The model under review builds one solid part; all positions refer to its coordinate system, in mm. Face numbers are marked on the shaded views. Round coordinates to 2 decimals unless told otherwise and drop trailing zeros. Order: outer loops, then holes, each group sorted by start corner. A loop starts at its lowest first (then second) coordinate and runs counter-clockwise, first axis right, second up. Notation, with made-up numbers: (-33, 31.25) -> (5, 31.25) arc R12 cw to (5, 53.25) -> close; hole circle Ø11 at (13, 86.25). An arc over 180 degrees is marked (long way). Use a Markdown table: item, result. Add a question column.
```python
from build123d import *

# Parameters (mm, degrees)
SKETCH_1_R               = 25
EXTRUDE_2_DEPTH          = 1
SKETCH_2_R               = 1.5
CUT_EXTRUDE_1_DEPTH      = 1
PATTERN_CIRCULAR_1_COUNT = 8
CUT_EXTRUDE_2_DEPTH      = 1
EXTRUDE_3_DEPTH          = 1
SKETCH_5_R               = 25
EXTRUDE_5_DEPTH          = 2
SKETCH_6_R               = 1.5
CUT_EXTRUDE_3_DEPTH      = 2
PATTERN_CIRCULAR_2_COUNT = 8
SKETCH_7_R               = 25
EXTRUDE_6_DEPTH          = 2
SKETCH_8_R               = 2.75
CUT_EXTRUDE_4_DEPTH      = 2
PATTERN_CIRCULAR_3_COUNT = 8
EXTRUDE_8_DEPTH          = 2


with BuildPart() as part:
    # 草图1 → 凸台-拉伸2 (new body)
    with BuildSketch(Plane(origin=(0, 0, 0), x_dir=(1, 0, 0), z_dir=(0, 1, 0))):
        Circle(SKETCH_1_R)
    extrude(amount=EXTRUDE_2_DEPTH)

    # 草图2 → 切除-拉伸1 (cut)
    with BuildSketch(Plane(origin=(0, 1, 0), x_dir=(1, 0, 0), z_dir=(0, 1, 0))):
        with Locations((18, 0)):
            Circle(SKETCH_2_R)
    cut_extrude_1 = extrude(amount=-CUT_EXTRUDE_1_DEPTH, mode=Mode.SUBTRACT)

    # 阵列(圆周)1: 切除-拉伸1 ×8 about axis
    pattern_circular_1_axis = Axis((0, 0, 0), (0, 1, 0))
    for i in range(1, PATTERN_CIRCULAR_1_COUNT):
        add(cut_extrude_1.rotate(pattern_circular_1_axis, i * 360 / PATTERN_CIRCULAR_1_COUNT), mode=Mode.SUBTRACT)

    # 草图3 → 切除-拉伸2 (cut)
    with BuildSketch(Plane(origin=(0, 1, 0), x_dir=(1, 0, 0), z_dir=(0, 1, 0))):
        Polygon((-15.202795796, 0), (15.202795796, 0), (0, -15.202795796), align=None)
    extrude(amount=-CUT_EXTRUDE_2_DEPTH, mode=Mode.SUBTRACT)

    # 草图4 → 凸台-拉伸3 (add)
    with BuildSketch(Plane(origin=(0, 1, 0), x_dir=(1, 0, 0), z_dir=(0, 1, 0))):
        Polygon((0, -14.849242405), (14.849242405, 0), (15.202795796, 0), (0, -15.202795796), (-15.202795796, 0), (-14.849242405, 0), align=None)
    extrude(amount=-EXTRUDE_3_DEPTH)

    # 草图5 → 凸台-拉伸5 (add)
    with BuildSketch(Plane.XZ):
        Circle(SKETCH_5_R)
    extrude(amount=EXTRUDE_5_DEPTH)

    # 草图6 → 切除-拉伸3 (cut)
    with BuildSketch(Plane(origin=(0, 0, 0), x_dir=(1, 0, 0), z_dir=(0, 1, 0))):
        with Locations((18, 0)):
            Circle(SKETCH_6_R)
    cut_extrude_3 = extrude(amount=-CUT_EXTRUDE_3_DEPTH, mode=Mode.SUBTRACT)

    # 阵列(圆周)2: 切除-拉伸3 ×8 about axis
    pattern_circular_2_axis = Axis((0, 1, 0), (0, -1, 0))
    for i in range(1, PATTERN_CIRCULAR_2_COUNT):
        add(cut_extrude_3.rotate(pattern_circular_2_axis, i * 360 / PATTERN_CIRCULAR_2_COUNT), mode=Mode.SUBTRACT)

    # 草图7 → 凸台-拉伸6 (add)
    with BuildSketch(Plane(origin=(0, 1, 0), x_dir=(1, 0, 0), z_dir=(0, 1, 0))):
        Circle(SKETCH_7_R)
        Polygon((-14.849242405, 0), (14.849242405, 0), (0, -14.849242405), align=None, mode=Mode.SUBTRACT)
    extrude(amount=EXTRUDE_6_DEPTH)

    # 草图8 → 切除-拉伸4 (cut)
    with BuildSketch(Plane(origin=(0, 1, 0), x_dir=(1, 0, 0), z_dir=(0, 1, 0))):
        with Locations((18, 0)):
            Circle(SKETCH_8_R)
    cut_extrude_4 = extrude(amount=CUT_EXTRUDE_4_DEPTH, mode=Mode.SUBTRACT)

    # 阵列(圆周)3: 切除-拉伸4 ×8 about axis
    pattern_circular_3_axis = Axis((0, 0, 0), (0, 1, 0))
    for i in range(1, PATTERN_CIRCULAR_3_COUNT):
        add(cut_extrude_4.rotate(pattern_circular_3_axis, i * 360 / PATTERN_CIRCULAR_3_COUNT), mode=Mode.SUBTRACT)

    # 草图9 → 凸台-拉伸8 (add)
    with BuildSketch(Plane(origin=(0, 0, 0), x_dir=(1, 0, 0), z_dir=(0, 1, 0))):
        Polygon((-14.849242405, 0), (14.849242405, 0), (0, -14.849242405), align=None)
    extrude(amount=EXTRUDE_8_DEPTH)


solid = part.part
```
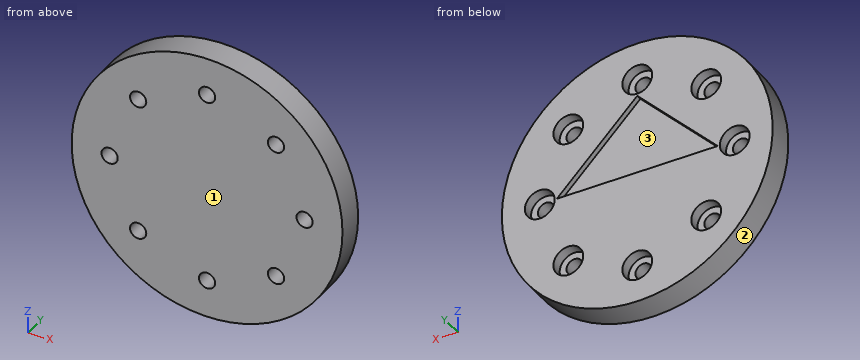
Q1. Add section A-A (x = -18). Write out the cut boundary in (y, z), then the cut area to 3 significant figures.
Q2. Add section B-B (z = 18). Write out the cut boundary in (x, y).
Q3. Mouldability with a two-part tool opening along X and no side actions: class the marked faces 1, 2 and 3 as pulls with the +X half, pulls with the -X half, needs draft (parallel to the pull), parting line crosses it, or undercut.
Q4. Insertion check: pin 1 (3.5 mm diameter, centred on x = 18, z = 0, fed in from +Y); pin 2 (3 mm diameter, centred on x = -10, y = 1, fed in from +Z). Each pin has a flat end and moves straight along its axis. Give the tip position at first contact, or say it passes through.
Q5. Add section C-C (y = -1.1). State how many separate pieces and enclosed holes the cut face has, then the cut area to 3 significant figures.
Q6. Wall thickness on line 1 (Z direction, x = 14.5, y = 1.45) (3 decimals); line 2 (Z direction, x = -13, y = -1.55); line 3 (X direction, y = 1.95, z = 1): over which ranges is each line inside the solid? List them lowest first. Write a range as [from, to].
Report:
| question | item | result |
|---|---|---|
| 1 | outline | (-2, -17.35) -> (3, -17.35) -> (3, -2.75) -> (1, -2.75) -> (1, -1.5) -> (-2, -1.5) -> close; (-2, 1.5) -> (1, 1.5) -> (1, 2.75) -> (3, 2.75) -> (3, 17.35) -> (-2, 17.35) -> close |
| 1 | area | 153 mm² |
| 2 | outline | (-17.35, -2) -> (-1.5, -2) -> (-1.5, 1) -> (-2.75, 1) -> (-2.75, 3) -> (-17.35, 3) -> close; (1.5, -2) -> (17.35, -2) -> (17.35, 3) -> (2.75, 3) -> (2.75, 1) -> (1.5, 1) -> close |
| 3 | face 1 | needs draft |
| 3 | face 2 | parting line crosses it |
| 3 | face 3 | undercut |
| 4 | pin 1 | stops at y = 1 |
| 4 | pin 2 | stops at z = 23.51 |
| 5 | separate pieces | 1 |
| 5 | enclosed holes | 8 |
| 5 | area | 1,910 mm² |
| 6 | line 1 | z = [-20.365, -14.831], [-10.625, 10.625], [14.831, 20.365] |
| 6 | line 2 | z = [-21.35, -14.2], [-11.25, 11.25], [14.2, 21.35] |
| 6 | line 3 | x = [-24.98, -20.56], [-15.44, 15.44], [20.56, 24.98] |
